Geometry check sheet. Reference: the model listing, model coordinates, mm. A direction names the side the tool comes from. Give positions to 0.01 mm unless a question says otherwise; leave off trailing zeros. Write each loop counter-clockwise with the first axis right and the second up, starting at its lowest first coordinate (ties: lowest second). Pieces come first, ordered by that corner, then holes.
(1) Depth check by flat-ended pin: P1, Ø3, axis at y = 7.5, z = 6.5, coming from the +X side. Enter the tip coordinate at first touch or a pass-through.
(2) Tool access check on faces 1 (the flat face through (-8, 10.5, 6)), 2 (the flat face through (0, 11, 10)). Record the directions out of +Z, -Z, +X, -X, +Y, -Y that give a thin tool (end or side, any length) a straight path to the whole face; none if there is none.
(3) Cross-section at D-D (y = 2.5). Record the boundary of the cut face in (x, z).
(4) Cross-section at C-C (z = 6). Record the boundary of the cut face in (x, y).
(5) Cross-section at A-A (x = -2.7). Record the boundary of the cut face in (y, z).
(6) Thickness scan on line 1 along Y through (x, z) = (-10.5, 0.5); line 2 along Z through (x, y) = (-2.7, -1.5); line 3 along X through (y, z) = (9.25, 0.75). Record the ranges inside material, lowest first.
(7) Cross-section at B-B (x = -7). Record the boundary of the cut face in (y, z), and give its area (3 significant figures).
(8) Mould release check, pull along Y, two halves, no side actions. Record for faces 3 (the flat face through (-7, 0, 6)), 4 (the flat face through (-12.4, 5.3, 0)), 5 (the flat face through (-9, -2, 6)): +Y half, -Y half, draft (parallel to the pull), parting line (faces both ways), or undercut.
```python
from build123d import *

# Parameters (mm, degrees)
F1_DEPTH = 12
F3_DEPTH = 33


with BuildPart() as f1:
    # F0 (on Top) → F1 (new body)
    with BuildSketch(Plane.XY):
        Polygon((0, -2), (0, 0), (-12.2, 0), (-12.2, 10.5), (0, 10.5), (0, 12.5), (-14.2, 12.5), (-14.2, -2), align=None)
    extrude(amount=F1_DEPTH)

    # F2 (on face) → F3 (cut, symmetric)
    with BuildSketch(Plane.XZ.offset(2)):
        with BuildLine():
            Line((0, 4.69233), (0, 7.30767))
            ThreePointArc((0, 7.30767), (-5.7, 6), (0, 4.69233))
        make_face()
    extrude(amount=F3_DEPTH, both=True, mode=Mode.SUBTRACT)


solid = f1.part
```
Reply:
1. P1: stops at x = -12.2
2. face 1: +Z, -Z, +X
2. face 2: +Z, -Z, +X, +Y, -Y
3. outline: (-14.2, 0) - (-12.2, 0) - (-12.2, 12) - (-14.2, 12) - close
4. outline: (-14.2, -2) - (-5.7, -2) - (-5.7, 0) - (-12.2, 0) - (-12.2, 10.5) - (-5.7, 10.5) - (-5.7, 12.5) - (-14.2, 12.5) - close
5. outline: (-2, 0) - (0, 0) - (0, 3) - (-2, 3) - close; (-2, 9) - (0, 9) - (0, 12) - (-2, 12) - close; (10.5, 0) - (12.5, 0) - (12.5, 3) - (10.5, 3) - close; (10.5, 9) - (12.5, 9) - (12.5, 12) - (10.5, 12) - close
6. line 1: y = -2 to 0, 10.5 to 12.5
6. line 2: z = 0 to 3, 9 to 12
6. line 3: x = -14.2 to -12.2
7. outline: (-2, 0) - (0, 0) - (0, 12) - (-2, 12) - close; (10.5, 0) - (12.5, 0) - (12.5, 12) - (10.5, 12) - close
7. area: 48.0 mm2
8. face 3: undercut
8. face 4: draft
8. face 5: -Y half
